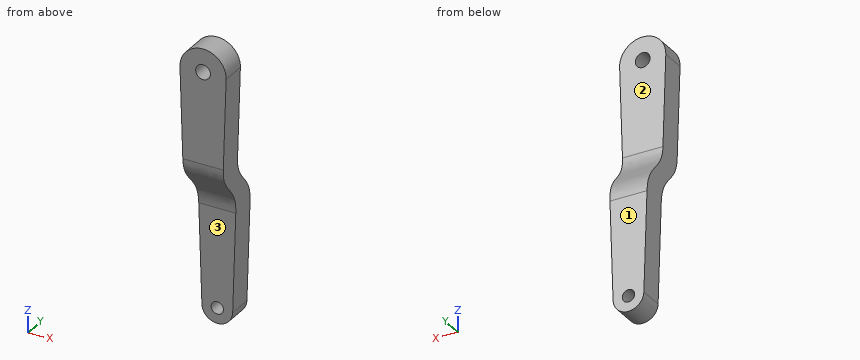
```python
from build123d import *

# Parameters (mm, degrees)
SKETCH1_R               = 1.2
SKETCH1_R_2             = 1
BOSS_EXTRUDE1_DEPTH     = 8
CUT_EXTRUDE7_DEPTH      = 44.408668489
CUT_EXTRUDE7_DEPTH_BACK = 44.408668489


with BuildPart() as part:
    # Sketch1 → Boss-Extrude1 (new body)
    with BuildSketch(Plane(origin=(0, 0, 0), x_dir=(1, 0, 0), z_dir=(0, 1, 0))):
        with BuildLine():
            ThreePointArc((-3.748168498, 0.1171875), (0, -3.75), (3.748168498, 0.1171875))
            Line((3.748168498, 0.1171875), (2.498778999, 40.078125))
            ThreePointArc((2.498778999, 40.078125), (0, 42.5), (-2.498778999, 40.078125))
            Line((-2.498778999, 40.078125), (-3.748168498, 0.1171875))
        make_face()
        with Locations(Location((0, 0, 0), (0, 0, 270))):
            Circle(SKETCH1_R, mode=Mode.SUBTRACT)
        with Locations(Location((0, 40, 0), (0, 0, 270))):
            Circle(SKETCH1_R_2, mode=Mode.SUBTRACT)
    extrude(amount=BOSS_EXTRUDE1_DEPTH)

    # Sketch4 → Cut-Extrude7 (cut, two sides: drawn at the far end of the back side and taken through both)
    with BuildSketch(Plane(origin=(0, 0, 0), x_dir=(0, 0, -1), z_dir=(1, 0, 0)).offset(-CUT_EXTRUDE7_DEPTH_BACK)):
        with BuildLine():
            Line((42.5, 4), (23.875, 4))
            add(Edge.make_bspline(
                [(14.875, 0), (19.125, 0), (19.123406576, 3.999999238), (23.875, 4)],
                knots=[0, 0, 0, 0, 1, 1, 1, 1], degree=3))
            ThreePointArc((14.875, 0), (31.025432495, -14.146346291), (42.5, 4))
        make_face()
        with BuildLine():
            Line((14.875, 4), (-3.75, 4))
            ThreePointArc((-3.75, 4), (8.0625, 19.8125), (23.875, 8))
            add(Edge.make_bspline(
                [(14.875, 4), (19.125, 4), (19.123406576, 7.999999238), (23.875, 8)],
                knots=[0, 0, 0, 0, 1, 1, 1, 1], degree=3))
        make_face()
    extrude(amount=CUT_EXTRUDE7_DEPTH + CUT_EXTRUDE7_DEPTH_BACK, mode=Mode.SUBTRACT)


solid = part.part
```
Read the model definition and answer for the solid it produces. Units are mm, in the model's axes. Face numbers are marked on the shaded views. A direction names the side the tool comes from. Coordinates: 2 decimals unless noted, no trailing zeros. Write each loop counter-clockwise with the first axis right and the second up, starting at its lowest first coordinate (ties: lowest second). Pieces come first, ordered by that corner, then holes. Notation, with made-up numbers: (52.25, 49.25) -> (110.25, 49.25) arc R15 ccw to (110.25, 76.25) -> close; hole circle Ø5 at (66.25, 85.5). An arc over 180 degrees is marked (long way). Return JSON: item names as keys, results as strings.
1. A cutting plane is placed at A-A (x = 0). Give the number of separate pieces and of enclosed holes in the cut face, and give its area (3 significant figures).
Found:
{"separate pieces": "3", "enclosed holes": "0", "area": "167 mm2"}
2. A cutting plane is placed at B-B (z = -6). Determine the outline of the cut face in (x, y).
Found:
{"outline": "(-3.56, 0) -> (3.56, 0) -> (3.56, 4) -> (-3.56, 4) -> close"}
3. A tool of negligible diameter and unlimited length cuts with its end or side. For the marked faces 1, 2 and 3, from which of +Z, -Z, +X, -X, +Y, -Y can it reach the whole face along a straight path? Write none if from no direction.
Found:
{"face 1": "+Z, -Z, +X, -X, +Y", "face 2": "+Z, +X, -X, +Y", "face 3": "-Z, +X, -X, -Y"}
4. Each of these flat-tipped pins is pushed along its axis until it touches: P1, Ø1.6, axis at x = 0, z = -40, coming from the -Y side; P2, Ø1, axis at x = 2, z = -14, coming from the +Y side; P3, Ø1.5, axis at x = 1.5, y = 1.5, coming from the +Z side. Where does it stop, or does it pass through?
Found:
{"P1": "through", "P2": "y = 4", "P3": "z = 3.67"}
5. Find the intervals of material crossed by line 1 along X through (y, z) = (5.1, -40); line 2 along Y through (x, z) = (-1.75, -1); line 3 along Z through (x, y) = (0, 5.05), in increasing order. Write a range as from..to.
Found:
{"line 1": "-2.5..-1, 1..2.5", "line 2": "0..4", "line 3": "-42.5..-41, -39..-18.06"}
